from build123d import *

# Parameters (mm, degrees)
SKETCH1_W               = 30.95625
SKETCH1_H               = 88.9
BOSS_EXTRUDE1_DEPTH     = 1.524
FILLET1_R               = 6.35
SKETCH6_R               = 1.524
CUT_EXTRUDE1_DEPTH      = 2.524
F_4_40_TAPPED_HOLE1_D   = 2.2606
F_1_2_13_TAPPED_HOLE1_D = 10.71626


with BuildPart() as part:
    # Sketch1 → Boss-Extrude1 (new body)
    with BuildSketch(Plane(origin=(0, 0, 0), x_dir=(1, 0, 0), z_dir=(0, 1, 0))):
        Rectangle(SKETCH1_W, SKETCH1_H)
    extrude(amount=BOSS_EXTRUDE1_DEPTH)

    # Fillet1
    fillet1_edges = [part.edges().sort_by_distance(p)[0] for p in [
        (15.478125, 0.762, -44.45),
        (15.478125, 0.762, 44.45),
        (-15.478125, 0.762, 44.45),
        (-15.478125, 0.762, -44.45),
    ]]
    fillet(fillet1_edges, radius=FILLET1_R)

    # Sketch6 → Cut-Extrude1 (cut, through all)
    with BuildSketch(Plane.XZ):
        with Locations((0, 14.478)):
            Circle(SKETCH6_R)
        with Locations((0, -14.478)):
            Circle(SKETCH6_R)
    extrude(amount=-CUT_EXTRUDE1_DEPTH, mode=Mode.SUBTRACT)

    # #4-40 Tapped Hole1 (through all)
    with Locations(Plane(origin=(0, 1.524, 0), x_dir=(-1, 0, 0), z_dir=(0, 1, 0))):
        with Locations((0, 25.4), (0, -25.4)):
            Hole(F_4_40_TAPPED_HOLE1_D / 2)

    # 1/2-13 Tapped Hole1 (through all)
    with Locations(Plane(origin=(0, 1.524, 0), x_dir=(-1, 0, 0), z_dir=(0, 1, 0))):
        with Locations((0, 0)):
            Hole(F_1_2_13_TAPPED_HOLE1_D / 2)


solid = part.part
Read the model definition and answer for the solid it produces. Units are mm, in the model's axes. Give positions to 0.01 mm unless a question says otherwise; leave off trailing zeros. Write each loop counter-clockwise with the first axis right and the second up, starting at its lowest first coordinate (ties: lowest second). Pieces come first, ordered by that corner, then holes. Notation, with made-up numbers: (-2.75, -33) -> (34.25, -33) arc R31 cw to (34.25, 4) -> close; hole circle Ø8 at (-27.5, 88.5). An arc over 180 degrees is marked (long way). Answer as a JSON object with one key per item and string values. Group by question number.
1) The mould has two halves that part along Z. Classify faces 1 (the cylindrical face through (13.67, 0.77, -42.54)), 2 (the flat face through (15.478, 1, 1)), 3 (the cylindrical face through (0.522, 0.751, -26.403)), 4 (the cylindrical face through (-13.67, 0.77, 42.54)): +Z half, -Z half, draft (parallel to the pull), parting line (faces both ways), or undercut.
2) Find section D-D (z = 25.4). Write down the section's boundary in (x, y).
3) Consider L1, parallel to Z at x = 0, y = 0.8; L2, parallel to X at y = 0.9, z = 25.5; L3, parallel to X at y = 1.45, z = 14. Determine where each line is inside the solid, lowest interval first. Write a range as from..to.
4) Find section A-A (x = 0). Write down the section's boundary in (y, z).
5) Find section C-C (y = 0.6). Write down the section's boundary in (x, z), and give its area (3 significant figures).
6) Find section B-B (z = 0). Write down the section's boundary in (x, y), and give its area (3 significant figures).
Values follow:
{
 "1": {"face 1": "-Z half", "face 2": "draft", "face 3": "undercut", "face 4": "+Z half"},
 "2": {"outline": "(-15.48, 0) -> (-1.13, 0) -> (-1.13, 1.52) -> (-15.48, 1.52) -> close; (1.13, 0) -> (15.48, 0) -> (15.48, 1.52) -> (1.13, 1.52) -> close"},
 "3": {"L1": "z = -44.45..-26.53, -24.27..-16, -12.95..-5.36, 5.36..12.95, 16..24.27, 26.53..44.45", "L2": "x = -15.48..-1.13, 1.13..15.48", "L3": "x = -15.48..-1.45, 1.45..15.48"},
 "4": {"outline": "(0, -44.45) -> (1.52, -44.45) -> (1.52, -26.53) -> (0, -26.53) -> close; (0, -24.27) -> (1.52, -24.27) -> (1.52, -16) -> (0, -16) -> close; (0, -12.95) -> (1.52, -12.95) -> (1.52, -5.36) -> (0, -5.36) -> close; (0, 5.36) -> (1.52, 5.36) -> (1.52, 12.95) -> (0, 12.95) -> close; (0, 16) -> (1.52, 16) -> (1.52, 24.27) -> (0, 24.27) -> close; (0, 26.53) -> (1.52, 26.53) -> (1.52, 44.45) -> (0, 44.45) -> close"},
 "5": {"outline": "(-15.48, -38.1) arc R6.35 ccw to (-9.13, -44.45) -> (9.13, -44.45) arc R6.35 ccw to (15.48, -38.1) -> (15.48, 38.1) arc R6.35 ccw to (9.13, 44.45) -> (-9.13, 44.45) arc R6.35 ccw to (-15.48, 38.1) -> close; hole circle Ø10.72 at (0, 0); hole circle Ø3.05 at (0, -14.48); hole circle Ø3.05 at (0, 14.48); hole circle Ø2.26 at (0, -25.4); hole circle Ø2.26 at (0, 25.4)", "area": "2,600 mm2"},
 "6": {"outline": "(-15.48, 0) -> (-5.36, 0) -> (-5.36, 1.52) -> (-15.48, 1.52) -> close; (5.36, 0) -> (15.48, 0) -> (15.48, 1.52) -> (5.36, 1.52) -> close", "area": "30.8 mm2"}
}
